from build123d import *

# Parameters (mm, degrees)
PAD_DEPTH        = 5
HOLE_D           = 6
HOLE_DEPTH       = 25
HOLE_CSINK_D     = 12
HOLE_CSINK_ANGLE = 90


with BuildPart() as part:
    # Sketch → Pad (new body)
    with BuildSketch(Plane.XY):
        Polygon((-200, 130), (200, 130), (200, 90), (45, 90), (45, 20), (200, 20), (200, -20), (45, -20), (45, -90), (200, -90), (200, -130), (-200, -130), (-200, -90), (-45, -90), (-45, -20), (-200, -20), (-200, 20), (-45, 20), (-45, 90), (-200, 90), align=None)
    extrude(amount=PAD_DEPTH)

    # Hole
    with Locations(Plane.XY.offset(5)):
        with Locations((0, 0), (0, 50), (0, 100), (0, -50), (0, -100)):
            CounterSinkHole(HOLE_D / 2, HOLE_CSINK_D / 2, depth=HOLE_DEPTH, counter_sink_angle=HOLE_CSINK_ANGLE)


solid = part.part
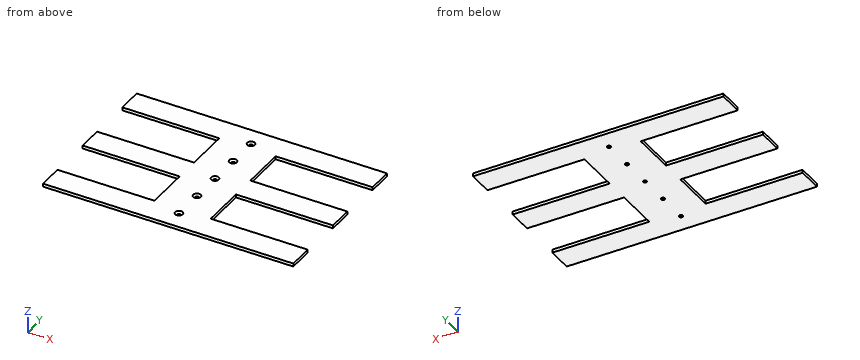
The model under review builds one solid part; all positions refer to its coordinate system, in mm. Round coordinates to 2 decimals unless told otherwise and drop trailing zeros. Loops run counter-clockwise (first coordinate to the right, second up) from the corner with the lowest first, then second, coordinate; pieces in that order, holes last. Notation, with made-up numbers: (23.5, -3.5) -> (49.5, -3.5) arc R18 cw to (49.5, 7.5) -> close; hole circle Ø6 at (5, 52). An arc over 180 degrees is marked (long way). Return JSON: item names as keys, results as strings.
(1) For line 1 (Y direction, x = -127, z = 1.5); line 2 (Y direction, x = 0, z = 1.3); line 3 (X direction, y = -50, z = 0.6), list the stretches that pass through material, from the lowest coordinate up.
Solved:
{"line 1": "-130 to -90, -20 to 20, 90 to 130", "line 2": "-130 to -103, -97 to -53, -47 to -3, 3 to 47, 53 to 97, 103 to 130", "line 3": "-45 to -3, 3 to 45"}
(2) Add section A-A on x = 163. Write out the cut boundary in (y, z), plus the area to 3 significant figures.
Solved:
{"outline": "(-130, 0) -> (-90, 0) -> (-90, 5) -> (-130, 5) -> close; (-20, 0) -> (20, 0) -> (20, 5) -> (-20, 5) -> close; (90, 0) -> (130, 0) -> (130, 5) -> (90, 5) -> close", "area": "600 mm2"}
(3) Add section C-C on y = -77.5. Write out the cut boundary in (x, z).
Solved:
{"outline": "(-45, 0) -> (45, 0) -> (45, 5) -> (-45, 5) -> close"}
(4) Add section B-B on z = 3.3. Write out the cut boundary in (x, y), plus the area to 3 significant figures.
Solved:
{"outline": "(-200, -130) -> (200, -130) -> (200, -90) -> (45, -90) -> (45, -20) -> (200, -20) -> (200, 20) -> (45, 20) -> (45, 90) -> (200, 90) -> (200, 130) -> (-200, 130) -> (-200, 90) -> (-45, 90) -> (-45, 20) -> (-200, 20) -> (-200, -20) -> (-45, -20) -> (-45, -90) -> (-200, -90) -> close; hole circle Ø8.6 at (0, -100); hole circle Ø8.6 at (0, -50); hole circle Ø8.6 at (0, 0); hole circle Ø8.6 at (0, 50); hole circle Ø8.6 at (0, 100)", "area": "60,300 mm2"}
(5) For pin 1 (1.5 mm diameter, centred on y = -43.5, z = 1.5, fed in from -X); pin 2 (7 mm diameter, centred on x = 0, y = -50, fed in from +Z); pin 3 (9.5 mm diameter, centred on x = 0, y = 100, fed in from +Z); pin 4 (6 mm diameter, centred on x = -33.5, y = -7.5, fed in from -Z), all flat-tipped, find the tip position at first contact; note any pin that passes through.
Solved:
{"pin 1": "x = -45", "pin 2": "z = 2.5", "pin 3": "z = 3.75", "pin 4": "z = 0"}
